Source: CAD feature listing. Evaluate the final solid. Frame: model axes, mm. A direction names the side the tool comes from. Give positions to 0.01 mm unless a question says otherwise; leave off trailing zeros. Write each loop counter-clockwise with the first axis right and the second up, starting at its lowest first coordinate (ties: lowest second). Pieces come first, ordered by that corner, then holes. Notation, with made-up numbers: (-19, 26.25) -> (13, 26.25) arc R25 cw to (13, 51.25) -> close; hole circle Ø1 at (15.25, -9.75). An arc over 180 degrees is marked (long way). Answer as a JSON object with one key per item and string values. Group by question number.
Item 1: First-contact query: pin 1 Ø6.5 at (y, z) = (-34.925, 12.7) entering from +X; pin 2 Ø8.5 at (y, z) = (31.75, 12.7) entering from -X; pin 3 Ø9.5 at (y, z) = (-31.75, 12.7) entering from -X. Flat tips, straight axial feed; report the tip coordinate or a pass-through.
Item 2: Section query B-B on x = 35. Give the number of separate pieces and of enclosed holes in the cut face, plus the area to 3 significant figures.
Item 3: Section query A-A on z = 6.25. Return the cut outline in (x, y), plus the area to 3 significant figures.
Item 4: Pull-direction query (Z, two-part tool) for faces 6 (the face through (34, -27.94, 13)), 7 (the face through (24.7, 35.19, 12.06)), 8 (the face through (-1, -32, 25.4)); classes: pulls with the +Z half, pulls with the -Z half, needs draft (parallel to the pull), parting line crosses it, or undercut.
Item 5: Ray query, probe 1 along Y at (x, z) = (-33, 12.7); probe 2 along Y at (x, z) = (39.25, 12.7); probe 3 along Y at (x, z) = (15.5, 22.25). Return the intervals inside material, ascending. Write a range as from..to.
Item 6: Section query D-D on x = 25.5. Return the cut outline in (y, z) (3 decimals), plus the area to 3 significant figures.
Item 7: Access query for faces 1 (the face through (35.684, 31.579, 10.566)), 2 (the face through (16.51, 0, 3)), 3 (the face through (-14, 0, 5.08)), 4 (the face through (-44.45, -1, 4)), 5 (the face through (-35.68, 36.98, 11.54)). Directions: +Z, -Z, +X, -X, +Y, -Y. A direction counts if a zero-diameter tool reaches every point of the face in a straight line with its end or side. Return the directions, or none.
Item 8: Section query C-C on x = -12.7. Return the cut outline in (y, z), plus the area to 3 significant figures.
from build123d import *

# Parameters (mm, degrees)
SKETCH1_W                  = 88.9
SKETCH1_H                  = 88.9
EXTRUDE1_DEPTH             = 25.4
F_1_2_0_5_DIAMETER_HOLE1_D = 12.7
EXTRUDE5_DEPTH             = 20.32
SKETCH16_W                 = 27.94
SKETCH16_H                 = 55.88
EXTRUDE6_DEPTH             = 6.08
FILLET2_R                  = 6.35


with BuildPart() as part:
    # Sketch1 → Extrude1 (new body)
    with BuildSketch(Plane.XY):
        Rectangle(SKETCH1_W, SKETCH1_H)
    extrude(amount=EXTRUDE1_DEPTH)

    # Sketch3 → Tap Drill for 3/8-16 Tap2 (revolve, cut)
    with BuildSketch(Plane(origin=(44.45, 34.925, 12.7), x_dir=(0, 0, -1), z_dir=(0, 1, 0))):
        Polygon((0, 0), (0, 20.164665582), (3.96875, 17.78), (3.96875, 0), align=None)
    tap_drill_for_3_8_16_tap2 = revolve(axis=Axis((50.8, 34.925, 12.7), (-1, 0, 0)), mode=Mode.SUBTRACT)

    # Mirror1: Tap Drill for 3/8-16 Tap2 across plane
    add(tap_drill_for_3_8_16_tap2.mirror(Plane.ZX), mode=Mode.SUBTRACT)

    # 1/2 (0.5) Diameter Hole1 (through all)
    with Locations(Plane.XY.offset(25.4)):
        with Locations((-12.7, 31.75)):
            f_1_2_0_5_diameter_hole1 = Hole(F_1_2_0_5_DIAMETER_HOLE1_D / 2)

    # Mirror3: 1/2 (0.5) Diameter Hole1 across plane
    add(f_1_2_0_5_diameter_hole1.mirror(Plane.ZX), mode=Mode.SUBTRACT)

    # Sketch15 → Extrude5 (cut)
    with BuildSketch(Plane.XY.offset(25.4)):
        Polygon((-44.45, 0), (-44.45, 19.05), (16.51, 19.05), (16.51, 27.94), (44.45, 27.94), (44.45, 0), align=None)
    extrude5 = extrude(amount=-EXTRUDE5_DEPTH, mode=Mode.SUBTRACT)

    # Mirror4: Extrude5 across plane
    add(extrude5.mirror(Plane.ZX), mode=Mode.SUBTRACT)

    # Sketch16 → Extrude6 (cut, through all)
    with BuildSketch(Plane.XY.offset(5.08)):
        with Locations((30.48, 0)):
            Rectangle(SKETCH16_W, SKETCH16_H)
    extrude(amount=-EXTRUDE6_DEPTH, mode=Mode.SUBTRACT)

    # Fillet2
    fillet2_edges = [part.edges().sort_by_distance(p)[0] for p in [
        (16.51, 27.94, 12.7),
        (16.51, -27.94, 12.7),
    ]]
    fillet(fillet2_edges, radius=FILLET2_R)

    # Sketch18 → Tap Drill for 1/2-13 Tap2 (revolve, cut)
    with BuildSketch(Plane(origin=(-44.45, 31.75, 12.7), x_dir=(0, 0, 1), z_dir=(0, 1, 0))):
        Polygon((0, 0), (0, 20.999489309), (5.35813, 17.78), (5.35813, 0), align=None)
    tap_drill_for_1_2_13_tap2 = revolve(axis=Axis((-50.8, 31.75, 12.7), (1, 0, 0)), mode=Mode.SUBTRACT)

    # Mirror5: Tap Drill for 1/2-13 Tap2 across plane
    add(tap_drill_for_1_2_13_tap2.mirror(Plane.ZX), mode=Mode.SUBTRACT)


solid = part.part
Worked answers:
{
 "1": {"pin 1": "x = 26.24", "pin 2": "x = -26", "pin 3": "x = -26.3"},
 "2": {"separate pieces": "2", "enclosed holes": "2", "area": "740 mm^2"},
 "3": {"outline": "(-44.45, -44.45) -> (44.45, -44.45) -> (44.45, -27.94) -> (22.86, -27.94) arc R6.35 cw to (16.51, -21.59) -> (16.51, -19.05) -> (-44.45, -19.05) -> close; (-44.45, 19.05) -> (16.51, 19.05) -> (16.51, 21.59) arc R6.35 cw to (22.86, 27.94) -> (44.45, 27.94) -> (44.45, 44.45) -> (-44.45, 44.45) -> close; hole circle Ø12.7 at (-12.7, -31.75); hole circle Ø12.7 at (-12.7, 31.75)", "area": "3,780 mm^2"},
 "4": {"face 6": "needs draft", "face 7": "undercut", "face 8": "pulls with the +Z half"},
 "5": {"probe 1": "-44.45..-37.11, -26.39..-19.05, 19.05..26.39, 37.11..44.45", "probe 2": "-44.45..-38.89, -30.96..-27.94, 27.94..30.96, 38.89..44.45", "probe 3": "-44.45..-19.05, 19.05..44.45"},
 "6": {"outline": "(-44.45, 0) -> (-27.94, 0) -> (-27.94, 25.4) -> (-44.45, 25.4) -> close; (27.94, 0) -> (44.45, 0) -> (44.45, 25.4) -> (27.94, 25.4) -> close; hole circle Ø4.043 at (-34.925, 12.7); hole circle Ø4.043 at (34.925, 12.7)", "area": "813 mm^2"},
 "7": {"face 1": "+X", "face 2": "+Z, -Z, +X", "face 3": "+Z, +X, -X", "face 4": "+Z, -Z, -X, +Y, -Y", "face 5": "-X"},
 "8": {"outline": "(-44.45, 0) -> (-38.1, 0) -> (-38.1, 25.4) -> (-44.45, 25.4) -> close; (-25.4, 0) -> (25.4, 0) -> (25.4, 25.4) -> (19.05, 25.4) -> (19.05, 5.08) -> (-19.05, 5.08) -> (-19.05, 25.4) -> (-25.4, 25.4) -> close; (38.1, 0) -> (44.45, 0) -> (44.45, 25.4) -> (38.1, 25.4) -> close", "area": "839 mm^2"}
}
